Read the model definition and answer for the solid it produces. Units are mm, in the model's axes. A direction names the side the tool comes from. Coordinates: 2 decimals unless noted, no trailing zeros. Write each loop counter-clockwise with the first axis right and the second up, starting at its lowest first coordinate (ties: lowest second). Pieces come first, ordered by that corner, then holes. Notation, with made-up numbers: (-14, -36.5) -> (40, -36.5) arc R11 ccw to (40, -20.5) -> close; hole circle Ø3 at (12.25, -40). An arc over 180 degrees is marked (long way). Return JSON: item names as keys, results as strings.
from build123d import *

# Parameters (mm, degrees)
SKETCH1_W           = 46
SKETCH1_H           = 46
BOSS_EXTRUDE1_DEPTH = 4
SKETCH2_W           = 46
SKETCH2_H           = 4
BOSS_EXTRUDE2_DEPTH = 42
SKETCH3_W           = 2
SKETCH3_H           = 42
BOSS_EXTRUDE3_DEPTH = 42
CHAMFER1_SIZE       = 42
SKETCH4_R           = 11.25
CUT_EXTRUDE1_DEPTH  = 42
SKETCH5_R           = 1.5
CUT_EXTRUDE2_DEPTH  = 42
SKETCH7_W           = 4
SKETCH7_H           = 46
BOSS_EXTRUDE4_DEPTH = 8
SKETCH8_W           = 4
SKETCH8_H           = 46
BOSS_EXTRUDE5_DEPTH = 8
CHAMFER2_SIZE       = 2
SKETCH6_R           = 1.5
CUT_EXTRUDE3_DEPTH  = 42


with BuildPart() as part:
    # Sketch1 → Boss-Extrude1 (new body)
    with BuildSketch(Plane(origin=(0, 0, 0), x_dir=(1, 0, 0), z_dir=(0, 1, 0))):
        with Locations((23, 23)):
            Rectangle(SKETCH1_W, SKETCH1_H)
    extrude(amount=BOSS_EXTRUDE1_DEPTH)

    # Sketch2 → Boss-Extrude2 (add)
    with BuildSketch(Plane(origin=(0, 4, 0), x_dir=(1, 0, 0), z_dir=(0, 1, 0))):
        with Locations((23, 44)):
            Rectangle(SKETCH2_W, SKETCH2_H)
    extrude(amount=BOSS_EXTRUDE2_DEPTH)

    # Sketch3 → Boss-Extrude3 (add)
    with BuildSketch(Plane(origin=(0, 4, 0), x_dir=(1, 0, 0), z_dir=(0, 1, 0))):
        with Locations((1, 21)):
            Rectangle(SKETCH3_W, SKETCH3_H)
        with Locations((45, 21)):
            Rectangle(SKETCH3_W, SKETCH3_H)
    extrude(amount=BOSS_EXTRUDE3_DEPTH)

    # Chamfer1
    chamfer1_edges = [part.edges().sort_by_distance(p)[0] for p in [
        (45, 46, 0),
        (1, 46, 0),
    ]]
    chamfer(chamfer1_edges, length=CHAMFER1_SIZE)

    # Sketch4 → Cut-Extrude1 (cut)
    with BuildSketch(Plane(origin=(0, 4, 0), x_dir=(1, 0, 0), z_dir=(0, 1, 0))):
        with Locations(Location((23, 21, 0), (0, 0, 270))):
            Circle(SKETCH4_R)
    extrude(amount=-CUT_EXTRUDE1_DEPTH, mode=Mode.SUBTRACT)

    # Sketch5 → Cut-Extrude2 (cut)
    with BuildSketch(Plane(origin=(0, 4, 0), x_dir=(1, 0, 0), z_dir=(0, 1, 0))):
        with Locations(Location((7.5, 36.5, 0), (0, 0, 270))):
            Circle(SKETCH5_R)
        with Locations(Location((7.5, 5.5, 0), (0, 0, 270))):
            Circle(SKETCH5_R)
        with Locations(Location((38.5, 5.5, 0), (0, 0, 270))):
            Circle(SKETCH5_R)
        with Locations(Location((38.5, 36.5, 0), (0, 0, 270))):
            Circle(SKETCH5_R)
    extrude(amount=-CUT_EXTRUDE2_DEPTH, mode=Mode.SUBTRACT)

    # Sketch7 → Boss-Extrude4 (add)
    with BuildSketch(Plane.ZY):
        with Locations((-44, 23)):
            Rectangle(SKETCH7_W, SKETCH7_H)
    extrude(amount=BOSS_EXTRUDE4_DEPTH)

    # Sketch8 → Boss-Extrude5 (add)
    with BuildSketch(Plane(origin=(46, 0, 0), x_dir=(0, 0, -1), z_dir=(1, 0, 0))):
        with Locations((44, 23)):
            Rectangle(SKETCH8_W, SKETCH8_H)
    extrude(amount=BOSS_EXTRUDE5_DEPTH)

    # Chamfer2
    chamfer2_edges = [part.edges().sort_by_distance(p)[0] for p in [
        (54, 46, -44),
        (54, 0, -44),
        (-8, 0, -44),
        (-8, 46, -44),
    ]]
    chamfer(chamfer2_edges, length=CHAMFER2_SIZE)

    # Sketch6 → Cut-Extrude3 (cut)
    with BuildSketch(Plane.XY.offset(-42)):
        with Locations((-4, 42)):
            Circle(SKETCH6_R)
        with Locations((-4, 4)):
            Circle(SKETCH6_R)
        with Locations((50, 4)):
            Circle(SKETCH6_R)
        with Locations((50, 42)):
            Circle(SKETCH6_R)
    extrude(amount=-CUT_EXTRUDE3_DEPTH, mode=Mode.SUBTRACT)


solid = part.part
1. Flat-ended cylindrical pins translate along their axes: pin 1 Ø2 at (y, z) = (23, -19.5) entering from -X; pin 2 Ø2.5 at (x, z) = (38.5, -5.5) entering from -Y; pin 3 Ø4 at (x, y) = (-4, 4) entering from +Z; pin 4 Ø10 at (x, y) = (0, 10) entering from +Z. Find the tip coordinate at first contact, or state that the pin passes through.
Taken from the geometry:
{"pin 1": "stops at x = 0", "pin 2": "passes through", "pin 3": "stops at z = -42", "pin 4": "stops at z = -1"}
2. Consider L1, parallel to Y at x = -4, z = -45.2; L2, parallel to X at y = 2, z = -36.5; L3, parallel to X at y = 5, z = -22. Determine where each line is inside the solid, lowest interval first.
Taken from the geometry:
{"L1": "y = 0 to 2.5, 5.5 to 40.5, 43.5 to 46", "L2": "x = 0 to 6, 9 to 37, 40 to 46", "L3": "x = 0 to 2, 44 to 46"}
3. The part is cut by section A-A (y = 42). Determine the outline of the cut face in (x, z), then the cut area to 3 significant figures.
Taken from the geometry:
{"outline": "(-8, -46) -> (-5.5, -46) -> (-5.5, -42) -> (-8, -42) -> close; (-2.5, -46) -> (48.5, -46) -> (48.5, -42) -> (46, -42) -> (46, -38) -> (44, -38) -> (44, -42) -> (2, -42) -> (2, -38) -> (0, -38) -> (0, -42) -> (-2.5, -42) -> close; (51.5, -46) -> (54, -46) -> (54, -42) -> (51.5, -42) -> close", "area": "240 mm2"}
4. The part is cut by section B-B (z = -21). Determine the outline of the cut face in (x, y), then the cut area to 3 significant figures.
Taken from the geometry:
{"outline": "(0, 0) -> (11.75, 0) -> (11.75, 4) -> (2, 4) -> (2, 25) -> (0, 25) -> close; (34.25, 0) -> (46, 0) -> (46, 25) -> (44, 25) -> (44, 4) -> (34.25, 4) -> close", "area": "178 mm2"}
5. The part is cut by section D-D (x = -4). Determine the outline of the cut face in (y, z), then the cut area to 3 significant figures.
Taken from the geometry:
{"outline": "(0, -46) -> (2.5, -46) -> (2.5, -42) -> (0, -42) -> close; (5.5, -46) -> (40.5, -46) -> (40.5, -42) -> (5.5, -42) -> close; (43.5, -46) -> (46, -46) -> (46, -42) -> (43.5, -42) -> close", "area": "160 mm2"}
6. For a pull along X with two mould halves and no side action, classify faces 1 (the face through (54, 23, -44)), 2 (the face through (23, 46, -44)), 3 (the face through (13.02, 2.03, -15.81)) as +X half, -X half, draft (parallel to the pull), parting line (faces both ways), or undercut.
Taken from the geometry:
{"face 1": "+X half", "face 2": "draft", "face 3": "undercut"}
7. A tool of negligible diameter and unlimited length cuts with its end or side. For faces 4 (the face through (37.036, 2.028, -5.825)), 5 (the face through (23, 25, -42)), 6 (the face through (0, 18, -25)), from which of +Z, -Z, +X, -X, +Y, -Y can it reach the whole face along a straight path? Write none if from no direction.
Taken from the geometry:
{"face 4": "+Y, -Y", "face 5": "+Z, +Y", "face 6": "+Z, -X, +Y, -Y"}
8. The part is cut by section C-C (x = 23). Determine the outline of the cut face in (y, z), then the cut area to 3 significant figures.
Taken from the geometry:
{"outline": "(0, -46) -> (46, -46) -> (46, -42) -> (4, -42) -> (4, -32.25) -> (0, -32.25) -> close; (0, -9.75) -> (4, -9.75) -> (4, 0) -> (0, 0) -> close", "area": "262 mm2"}
